```python
from build123d import *

# Parameters (mm, degrees)
BOSS_EXTRU_1_DEPTH      = 90
ESQUISSE3_W             = 39
ESQUISSE3_H             = 9
ENL_V_MAT_EXTRU_1_DEPTH = 5
ESQUISSE4_R             = 1.25
ENL_V_MAT_EXTRU_2_DEPTH = 5
ESQUISSE5_W             = 39
ESQUISSE5_H             = 9
ENL_V_MAT_EXTRU_3_DEPTH = 16


with BuildPart() as part:
    # Esquisse1 → Boss.-Extru.1 (new body)
    with BuildSketch(Plane.XY):
        Polygon((0, 0), (-2, 0), (-2, 9), (-3, 9), (-3, 0), (-5, 0), (-5, 9), (-6, 9), (-6, 0), (-8, 0), (-8, 9), (-9, 9), (-9, 0), (-10, 0), (-10, 9), (-11, 9), (-11, 0), (-13, 0), (-13, 9), (-14, 9), (-14, 0), (-16, 0), (-16, 9), (-17, 9), (-17, 0), (-18, 0), (-18, 9), (-19, 9), (-19, 0), (-21, 0), (-21, 9), (-22, 9), (-22, 0), (-24, 0), (-24, 9), (-25, 9), (-25, 0), (-26, 0), (-26, 9), (-27, 9), (-27, 0), (-29, 0), (-29, 9), (-30, 9), (-30, 0), (-32, 0), (-32, 9), (-33, 9), (-33, 0), (-34, 0), (-34, 9), (-35, 9), (-35, 0), (-37, 0), (-37, 9), (-38, 9), (-38, 0), (-40, 0), (-40, 9), (-41, 9), (-41, 0), (-42, 0), (-42, 10), (0, 10), align=None)
    extrude(amount=BOSS_EXTRU_1_DEPTH)

    # Esquisse3 → Enlèv. mat.-Extru.1 (cut)
    with BuildSketch(Plane.XY.offset(90)):
        with Locations((-21.5, 4.5)):
            Rectangle(ESQUISSE3_W, ESQUISSE3_H)
    extrude(amount=-ENL_V_MAT_EXTRU_1_DEPTH, mode=Mode.SUBTRACT)

    # Esquisse4 → Enlèv. mat.-Extru.2 (cut)
    with BuildSketch(Plane(origin=(0, 10, 0), x_dir=(1, 0, 0), z_dir=(0, 1, 0))):
        with Locations(Location((-31, -87, 0), (0, 0, 270))):
            Circle(ESQUISSE4_R)
        with Locations(Location((-11, -87, 0), (0, 0, 270))):
            Circle(ESQUISSE4_R)
        with Locations(Location((-11, -13, 0), (0, 0, 90))):
            Circle(ESQUISSE4_R)
        with Locations(Location((-31, -13, 0), (0, 0, 323.130102354))):
            Circle(ESQUISSE4_R)
    extrude(amount=-ENL_V_MAT_EXTRU_2_DEPTH, mode=Mode.SUBTRACT)

    # Esquisse5 → Enlèv. mat.-Extru.3 (cut)
    with BuildSketch(Plane(origin=(0, 0, 0), x_dir=(-1, 0, 0), z_dir=(0, 0, -1))):
        with Locations((21.5, 4.5)):
            Rectangle(ESQUISSE5_W, ESQUISSE5_H)
    extrude(amount=-ENL_V_MAT_EXTRU_3_DEPTH, mode=Mode.SUBTRACT)


solid = part.part
```
Model file for the job. Use its own axes, mm. A direction names the side the tool comes from. Give positions to 0.01 mm unless a question says otherwise; leave off trailing zeros. Write each loop counter-clockwise with the first axis right and the second up, starting at its lowest first coordinate (ties: lowest second). Pieces come first, ordered by that corner, then holes. Notation, with made-up numbers: (42, 81.25) - (90, 81.25) arc R19 cw to (90, 93.25) - close; hole circle Ø5 at (21, 45). An arc over 180 degrees is marked (long way). One line per question, with ' | ' between items. Start each with the question number.
(1) Slice it at B-B on z = 87. Write the cut outline in (x, y), plus the area to 3 significant figures.
(2) Slice it at C-C on z = 10.5. Write the cut outline in (x, y).
(3) Wall check: line 1 along X through (y, z) = (9.45, 87); line 2 along X through (y, z) = (2.25, 5.5); line 3 along Z through (x, y) = (-6.5, 8.5). Give the ranges that are in metal, low to high. Write a range as from..to.
(4) Two-plate mould, pull along X, no slides. Class faces 1 (the face through (-23, 5, 16)), 2 (the face through (-20, 0, 50)): +X half, -X half, draft (parallel to the pull), parting line (faces both ways), or undercut.
(5) Pin check, flat tips, straight feed: P1, Ø0.6, axis at x = -31.5, y = 4, coming from the +Z side; P2, Ø3, axis at x = -11, z = 87, coming from the +Y side; P3, Ø2, axis at x = -27.5, y = 4.5, coming from the -Z side. Stop position of each tip, or through.
(6) 3-axis set-ups, long thin cutter, end or side, ignore diameter. For faces 3 (the face through (-31.97, 9.51, 12.21)), 4 (the face through (-36, 5, 16)), 5 (the face through (-20, 5, 85)), 6 (the face through (-5, 4, 50)): which of +Z, -Z, +X, -X, +Y, -Y reach the whole face in a straight line?
(7) Slice it at D-D on y = 2.5. Give the number of separate pieces and of enclosed holes in the cut face, plus the area to 3 significant figures.
(8) Slice it at A-A on x = -31. Write the cut outline in (y, z).
Results below:
1) outline: (-42, 0) - (-41, 0) - (-41, 9) - (-32.25, 9) - (-32.25, 10) - (-42, 10) - close; (-29.75, 9) - (-12.25, 9) - (-12.25, 10) - (-29.75, 10) - close; (-9.75, 9) - (-2, 9) - (-2, 0) - (0, 0) - (0, 10) - (-9.75, 10) - close | area: 64.0 mm^2
2) outline: (-42, 0) - (-41, 0) - (-41, 9) - (-2, 9) - (-2, 0) - (0, 0) - (0, 10) - (-42, 10) - close
3) line 1: -42..-32.25, -29.75..-12.25, -9.75..0 | line 2: -42..-41, -2..0 | line 3: 16..85
4) face 1: undercut | face 2: draft
5) P1: z = 85 | P2: y = 10 | P3: z = 16
6) face 3: +Y, -Y | face 4: -Z, -Y | face 5: +Z, -Y | face 6: +Z, -Z, -Y
7) separate pieces: 16 | enclosed holes: 0 | area: 1,930 mm^2
8) outline: (0, 16) - (9, 16) - (9, 14.25) - (10, 14.25) - (10, 85.75) - (9, 85.75) - (9, 85) - (0, 85) - close; (9, 0) - (10, 0) - (10, 11.75) - (9, 11.75) - close; (9, 88.25) - (10, 88.25) - (10, 90) - (9, 90) - close
